Geometry check sheet. Reference: the model listing, model coordinates, mm. Round coordinates to 2 decimals unless told otherwise and drop trailing zeros. Order: outer loops, then holes, each group sorted by start corner. A loop starts at its lowest first (then second) coordinate and runs counter-clockwise, first axis right, second up. Notation, with made-up numbers: (-27.5, 25) -> (-19.5, 25) arc R33 ccw to (-19.5, 61) -> close; hole circle Ø6 at (-36.5, 36.5). An arc over 180 degrees is marked (long way). Use a Markdown table: item, result. Add a question column.
Item 1: Material ranges on probe 1 along Y at (x, z) = (191, 2.6); probe 2 along Y at (x, z) = (496, 2.4); probe 3 along Y at (x, z) = (393.7, 1.15) (3 decimals), recorded low to high. Write a range as [from, to].
Item 2: Sectioned sample at C-C, the plane x = 254. Record the cut outline in (y, z) (3 decimals), and give its area (3 significant figures).
Item 3: Sectioned sample at A-A, the plane y = -115.5. Record the cut outline in (x, z) (3 decimals).
Item 4: Sectioned sample at D-D, the plane z = 2.4. State how many separate pieces and enclosed holes the cut face has, and give its area (3 significant figures).
Item 5: Sectioned sample at B-B, the plane x = 85.5. Record the cut outline in (y, z) (3 decimals).
from build123d import *

# Parameters (mm, degrees)
F0_R     = 2.1844
F0_R_2   = 14.2875
F0_W     = 50.8
F0_H     = 177.8
F0_W_2   = 196.85
F0_H_2   = 9.525
F1_DEPTH = 3.175


# Not quite as in the source:
# - a feature names something its author has since deleted; it is built from what else it names


with BuildPart() as f1:
    # F0 (on Top) → F1 (new body)
    with BuildSketch(Plane.XY):
        Polygon((431.8, 0), (0, 0), (0, -127), (127, -127), (127, -609.6), (0, -609.6), (0, -736.6), (431.8, -736.6), (431.8, -660.4), (482.6, -660.4), (482.6, -457.2), (584.2, -457.2), (584.2, -366.7125), (387.35, -366.7125), (387.35, -357.1875), (584.2, -357.1875), (584.2, -279.4), (482.6, -279.4), (482.6, -76.2), (431.8, -76.2), align=None)
        with Locations((139.7, -495.3)):
            Circle(F0_R, mode=Mode.SUBTRACT)
        with Locations((165.1, -495.3)):
            Circle(F0_R, mode=Mode.SUBTRACT)
        with Locations((254, -532.4475)):
            Circle(F0_R_2, mode=Mode.SUBTRACT)
        with Locations((190.5, -495.3)):
            Circle(F0_R, mode=Mode.SUBTRACT)
        with Locations((215.9, -495.3)):
            Circle(F0_R, mode=Mode.SUBTRACT)
        with Locations((241.3, -495.3)):
            Circle(F0_R, mode=Mode.SUBTRACT)
        with Locations((266.7, -495.3)):
            Circle(F0_R, mode=Mode.SUBTRACT)
        with Locations((292.1, -495.3)):
            Circle(F0_R, mode=Mode.SUBTRACT)
        with Locations((317.5, -495.3)):
            Circle(F0_R, mode=Mode.SUBTRACT)
        with Locations((342.9, -495.3)):
            Circle(F0_R, mode=Mode.SUBTRACT)
        Polygon((387.35, -498.475), (438.15, -498.475), (438.15, -568.325), (292.1, -568.325), (292.1, -498.475), align=None, mode=Mode.SUBTRACT)
        with Locations((368.3, -495.3)):
            Circle(F0_R, mode=Mode.SUBTRACT)
        with Locations((393.7, -495.3)):
            Circle(F0_R, mode=Mode.SUBTRACT)
        with Locations((419.1, -495.3)):
            Circle(F0_R, mode=Mode.SUBTRACT)
        with Locations((444.5, -495.3)):
            Circle(F0_R, mode=Mode.SUBTRACT)
        with Locations((469.9, -495.3)):
            Circle(F0_R, mode=Mode.SUBTRACT)
        with Locations((139.7, -241.3)):
            Circle(F0_R, mode=Mode.SUBTRACT)
        with Locations((165.1, -241.3)):
            Circle(F0_R, mode=Mode.SUBTRACT)
        with Locations((190.5, -241.3)):
            Circle(F0_R, mode=Mode.SUBTRACT)
        with Locations((215.9, -241.3)):
            Circle(F0_R, mode=Mode.SUBTRACT)
        with Locations((241.3, -241.3)):
            Circle(F0_R, mode=Mode.SUBTRACT)
        with Locations((266.7, -241.3)):
            Circle(F0_R, mode=Mode.SUBTRACT)
        with Locations((254, -191.4525)):
            Circle(F0_R_2, mode=Mode.SUBTRACT)
        with Locations((292.1, -241.3)):
            Circle(F0_R, mode=Mode.SUBTRACT)
        with Locations((317.5, -241.3)):
            Circle(F0_R, mode=Mode.SUBTRACT)
        with Locations((342.9, -241.3)):
            Circle(F0_R, mode=Mode.SUBTRACT)
        with Locations((368.3, -241.3)):
            Circle(F0_R, mode=Mode.SUBTRACT)
        with Locations((393.7, -241.3)):
            Circle(F0_R, mode=Mode.SUBTRACT)
        with Locations((419.1, -241.3)):
            Circle(F0_R, mode=Mode.SUBTRACT)
        with Locations((444.5, -241.3)):
            Circle(F0_R, mode=Mode.SUBTRACT)
        with Locations((469.9, -241.3)):
            Circle(F0_R, mode=Mode.SUBTRACT)
        Polygon((685.8, 0), (431.8, 0), (431.8, -76.2), (482.6, -76.2), (635, -76.2), (685.8, -76.2), align=None)
        Polygon((711.2, 0), (685.8, 0), (685.8, -76.2), (685.8, -254), (711.2, -254), align=None)
        with Locations((698.5, -241.3)):
            Circle(F0_R, mode=Mode.SUBTRACT)
        with Locations((660.4, -165.1)):
            Rectangle(F0_W, F0_H)
        with Locations((647.7, -241.3)):
            Circle(F0_R, mode=Mode.SUBTRACT)
        with Locations((673.1, -241.3)):
            Circle(F0_R, mode=Mode.SUBTRACT)
        Polygon((431.8, -660.4), (431.8, -736.6), (685.8, -736.6), (685.8, -660.4), (635, -660.4), (482.6, -660.4), align=None)
        Polygon((711.2, -736.6), (711.2, -482.6), (685.8, -482.6), (685.8, -660.4), (685.8, -736.6), align=None)
        with Locations((698.5, -495.3)):
            Circle(F0_R, mode=Mode.SUBTRACT)
        with Locations((660.4, -571.5)):
            Rectangle(F0_W, F0_H)
        with Locations((647.7, -495.3)):
            Circle(F0_R, mode=Mode.SUBTRACT)
        with Locations((673.1, -495.3)):
            Circle(F0_R, mode=Mode.SUBTRACT)
        with Locations((485.775, -361.95)):
            Rectangle(F0_W_2, F0_H_2)
    extrude(amount=F1_DEPTH)


solid = f1.part
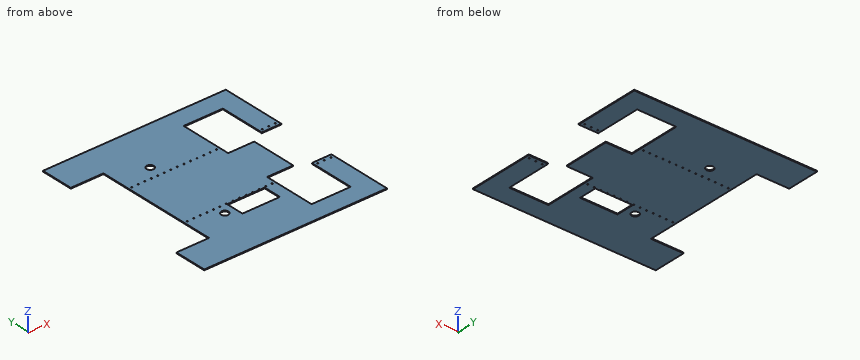
Found:
| question | item | result |
|---|---|---|
| 1 | probe 1 | y = [-736.6, -497.43], [-493.17, -243.43], [-239.17, 0] |
| 1 | probe 2 | y = [-736.6, -660.4], [-457.2, -279.4], [-76.2, 0] |
| 1 | probe 3 | y = [-736.6, -568.325], [-498.475, -497.484], [-493.116, -243.484], [-239.116, 0] |
| 2 | outline | (-736.6, 0) -> (-546.735, 0) -> (-546.735, 3.175) -> (-736.6, 3.175) -> close; (-518.16, 0) -> (-205.74, 0) -> (-205.74, 3.175) -> (-518.16, 3.175) -> close; (-177.165, 0) -> (0, 0) -> (0, 3.175) -> (-177.165, 3.175) -> close |
| 2 | area | 2,160 mm2 |
| 3 | outline | (0, 0) -> (482.6, 0) -> (482.6, 3.175) -> (0, 3.175) -> close; (635, 0) -> (711.2, 0) -> (711.2, 3.175) -> (635, 3.175) -> close |
| 4 | separate pieces | 1 |
| 4 | enclosed holes | 37 |
| 4 | area | 362,000 mm2 |
| 5 | outline | (-736.6, 0) -> (-609.6, 0) -> (-609.6, 3.175) -> (-736.6, 3.175) -> close; (-127, 0) -> (0, 0) -> (0, 3.175) -> (-127, 3.175) -> close |
